Could you check a few things on this model? Use its own coordinates, in mm. Coordinates: 2 decimals unless noted, no trailing zeros. Loops run counter-clockwise (first coordinate to the right, second up) from the corner with the lowest first, then second, coordinate; pieces in that order, holes last. Notation, with made-up numbers: M -8.75,85 L 19.25,85 A9 cw 19.25,100 Z; hole C 31.25,-20 d4. An arc over 180 degrees is marked long. Write each question's results on one line, items separated by ' | '.
Autodesk Inventor part; units mm, degrees
ref_plane "YZ Plane" through (0, 0, 0) normal (1, 0, 0) x (0, 1, 0)
ref_plane "XZ Plane" through (0, 0, 0) normal (0, 1, 0) x (-1, 0, 0)
ref_plane "XY Plane" through (0, 0, 0) normal (0, 0, 1) x (1, 0, 0)
sketch "Sketch1" plane through (0, 0, 0) normal (0, 0, 1) x (1, 0, 0)
  circle A0 centre (0, 0) radius 4
  circle A1 centre (-35, 0) radius 4
  line L0 (-35, 4) -> (0, 4)
  line L1 (0, -4) -> (-35, -4)
  dimension "d0" = 8
  dimension "d1" = 8
  dimension "d2" = 35
extrude "Extrusion1" add sketch "Sketch1" along normal blind 3
sketch "Sketch3" plane through (0, 0, 3) normal (0, 0, 1) x (1, 0, 0)
  arc A0 (-35, 4) -> (-35, -4) centre (-35, 0) ccw
  line L0 (-35, -4) -> (0, -4)
  arc A1 (0, -4) -> (0, 4) centre (0, 0) ccw
  line L1 (0, 4) -> (-35, 4)
hole "Hole1" at (0, 0, 3) direction (0, 0, -1) diameter 3 end through all
sketch "Sketch4" plane through (0, 0, 3) normal (0, 0, 1) x (1, 0, 0)
  circle A0 centre (0, 0) radius 1.5
  arc A1 (-35, 4) -> (-35, -4) centre (-35, 0) ccw
  line L0 (-35, -4) -> (0, -4)
  arc A2 (0, -4) -> (0, 4) centre (0, 0) ccw
  line L1 (0, 4) -> (-35, 4)
hole "Hole2" at (-35, 0, 3) direction (0, 0, -1) diameter 3.4 end through all
properties part number "Selection_Counterweight" material "Nylon 6/6"
(1) If we mould it in two halves opening along X, with no side actions, what happens to faces 1 (the cylindrical face through (4, 0, 1)), 2 (the cylindrical face through (-33.34, 0.37, 1.48)), 3 (the flat face through (-18, 4, 1)), 4 (the cylindrical face through (-0.07, 1.5, 1.48))? For each: released by +X, released by -X, zero draft, split by the parting line, or undercut.
Reported:
face 1: released by +X | face 2: undercut | face 3: zero draft | face 4: undercut
(2) Imagine slicing it at A-A, the plane y = 0. List the corners of the cut face in (x, z) for me.
Reported:
outline: M -39,0 L -36.7,0 L -36.7,3 L -39,3 Z; M -33.3,0 L -1.5,0 L -1.5,3 L -33.3,3 Z; M 1.5,0 L 4,0 L 4,3 L 1.5,3 Z
(3) Imagine slicing it at C-C, the plane y = -2.75. List the corners of the cut face in (x, z) for me.
Reported:
outline: M -37.9,0 L 2.9,0 L 2.9,3 L -37.9,3 Z
(4) Imagine slicing it at B-B, the plane z = 2.4. List the corners of the cut face in (x, y) for me.
Reported:
outline: M -35,-4 L 0,-4 A4 ccw 0,4 L -35,4 A4 ccw Z; hole C -35,0 d3.4; hole C 0,0 d3
(5) Will these pins go through, and if not, where does the flat tip stop? P1, Ø3, axis at x = -35, y = 0, coming from the -Z side; P2, Ø1, axis at y = 0.5, z = 2.5, coming from the -X side.
Reported:
P1: passes through | P2: stops at x = -39
(6) Please list where these lines run through material, in increasing order: probe 1 along X at (y, z) = (0, 2.35); probe 2 along Y at (x, z) = (0, 1.6); probe 3 along Y at (x, z) = (-35, 1). Write a range as from..to.
Reported:
probe 1: x = -39..-36.7, -33.3..-1.5, 1.5..4 | probe 2: y = -4..-1.5, 1.5..4 | probe 3: y = -4..-1.7, 1.7..4
